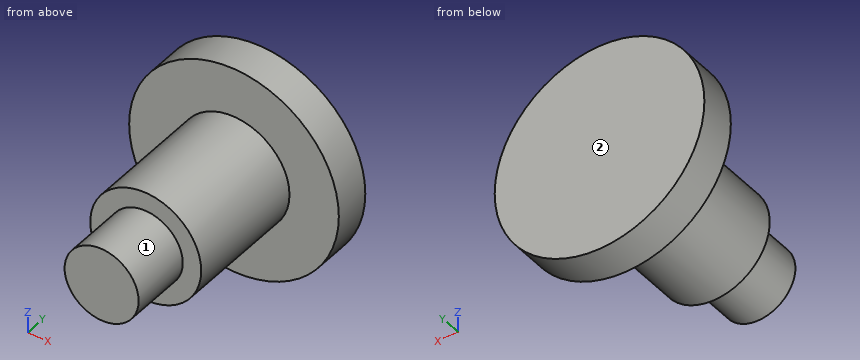
from build123d import *

# Parameters (mm, degrees)
SKETCH1_R           = 4.25
BOSS_EXTRUDE1_DEPTH = 1.5
SKETCH1_3_R         = 2.25
BOSS_EXTRUDE2_DEPTH = 5
SKETCH2_R           = 1.5
BOSS_EXTRUDE3_DEPTH = 2.5


with BuildPart() as part:
    # Sketch1 → Boss-Extrude1 (new body)
    with BuildSketch(Plane(origin=(0, 0, 0), x_dir=(1, 0, 0), z_dir=(0, 1, 0))):
        Circle(SKETCH1_R)
    extrude(amount=BOSS_EXTRUDE1_DEPTH)

    # Sketch1<3> → Boss-Extrude2 (add)
    with BuildSketch(Plane(origin=(0, 0, 0), x_dir=(1, 0, 0), z_dir=(0, 1, 0))):
        Circle(SKETCH1_3_R)
    extrude(amount=-BOSS_EXTRUDE2_DEPTH)

    # Sketch2 → Boss-Extrude3 (add)
    with BuildSketch(Plane.XZ.offset(5)):
        with Locations((0, -0.007534146)):
            Circle(SKETCH2_R)
    extrude(amount=BOSS_EXTRUDE3_DEPTH)


solid = part.part
Design review of the part built by this model. Coordinates are the model's own, in mm. Face numbers are marked on the shaded views. A direction names the side the tool comes from. Coordinates: 2 decimals unless noted, no trailing zeros. Write each loop counter-clockwise with the first axis right and the second up, starting at its lowest first coordinate (ties: lowest second). Pieces come first, ordered by that corner, then holes. Notation, with made-up numbers: (-24, 21.25) -> (16, 21.25) arc R21 ccw to (16, 44.25) -> close; hole circle Ø6 at (-31, 4). An arc over 180 degrees is marked (long way). Write each question's results on one line, items separated by ' | '. Start each with the question number.
(1) Tool access review of the marked faces 1 and 2: name each direction out of +Z, -Z, +X, -X, +Y, -Y from which nothing blocks a thin tool from reaching the whole face with its end or side.
(2) Take a section at D-D on z = 1.75. Write out the cut boundary in (x, y).
(3) For line 1 along Y through (x, z) = (3.25, -0.25); line 2 along X through (y, z) = (0.5, 1.25); line 3 along Y through (x, z) = (1.5, 1), list the stretches that pass through material, from the lowest coordinate up. Write a range as from..to.
(4) Clearance check with flat-ended pins moving along their axes: P1, Ø5, axis at x = -1.5, y = -5, coming from the +Z side; P2, Ø3, axis at y = -5, z = 2.5, coming from the -X side; P3, Ø4, axis at x = -3.5, y = -5.5, coming from the -Z side. State where each tip first meets the part, or that it passes through.
(5) Take a section at B-B on z = -0.5. Write out the cut boundary in (x, y).
(6) Take a section at A-A on x = 0. Write out the cut boundary in (y, z), and give its area (4 significant figures).
(7) Take a section at C-C on y = -0.5. Write out the cut boundary in (x, z), and give its area (3 significant figures).
Results found:
1) face 1: -Y | face 2: +Z, -Z, +X, -X, +Y
2) outline: (-3.87, 0) -> (-1.41, 0) -> (-1.41, -5) -> (1.41, -5) -> (1.41, 0) -> (3.87, 0) -> (3.87, 1.5) -> (-3.87, 1.5) -> close
3) line 1: y = 0..1.5 | line 2: x = -4.06..4.06 | line 3: y = -5..1.5
4) P1: stops at z = 2.25 | P2: stops at x = -2.02 | P3: stops at z = -1.62
5) outline: (-4.22, 0) -> (-2.19, 0) -> (-2.19, -5) -> (-1.42, -5) -> (-1.42, -7.5) -> (1.42, -7.5) -> (1.42, -5) -> (2.19, -5) -> (2.19, 0) -> (4.22, 0) -> (4.22, 1.5) -> (-4.22, 1.5) -> close
6) outline: (-7.5, -1.51) -> (-5, -1.51) -> (-5, -2.25) -> (0, -2.25) -> (0, -4.25) -> (1.5, -4.25) -> (1.5, 4.25) -> (0, 4.25) -> (0, 2.25) -> (-5, 2.25) -> (-5, 1.49) -> (-7.5, 1.49) -> close | area: 42.75 mm2
7) outline: circle Ø4.5 at (0, 0) | area: 15.9 mm2
